For this review, take the finished solid that the model builds, in its own axes (mm). A direction names the side the tool comes from. Coordinates: 2 decimals unless noted, no trailing zeros. Order: outer loops, then holes, each group sorted by start corner. A loop starts at its lowest first (then second) coordinate and runs counter-clockwise, first axis right, second up. Notation, with made-up numbers: (-22.5, 45) -> (-5.5, 45) arc R32 cw to (-5.5, 80) -> close; hole circle Ø10 at (74, 16). An arc over 180 degrees is marked (long way). Answer as a JSON object with one key per item and string values. Group by question number.
1) Machinability: for faces 1 (the flat face through (7, 0, 15)), 2 (the flat face through (-7, 0, 15)), 3 (the flat face through (0, -7, 15)), 4 (the flat face through (-0.1, 5.4, 0)), 5 (the flat face through (0, 0, 18)), which of the approach directions +Z, -Z, +X, -X, +Y, -Y give a long, thin tool a straight path to every point of the face, cutting with its end or side? Answer none if there is none.
2) Wall thickness on L1, parallel to X at y = -3.5, z = 6.25; L2, parallel to X at y = 3, z = 10.5: over which ranges is each line inside the solid? List them lowest first.
3) For pin 1 (8 mm diameter, centred on x = -4, y = 5, fed in from -Z); pin 2 (8 mm diameter, centred on x = -1.5, z = 14.5, fed in from +Y); pin 3 (1 mm diameter, centred on y = 1, z = 13.5, fed in from +X); pin 4 (3 mm diameter, centred on y = 2, z = 15.5, fed in from -X), all flat-tipped, find the tip position at first contact; note any pin that passes through.
4) Draft analysis for pull direction X (two halves, no side actions). For faces 6 (the flat face through (5, 0, 9)), 7 (the flat face through (-8, 0, 5)), 8 (the flat face through (0, 7, 15)), state which applies: +X half, -X half, draft (parallel to the pull), parting line (faces both ways), or undercut.
5) Add section D-D, the plane z = 17.25. Write out the cut boundary in (x, y), then the cut area to 3 significant figures.
6) Add section B-B, the plane x = 2.25. Write out the cut boundary in (y, z).
7) Add section A-A, the plane z = 8. Write out the cut boundary in (x, y), then the cut area to 3 significant figures.
from build123d import *

# Parameters (mm, degrees)
BOX002_W     = 10
BOX002_H     = 10
BOX002_DEPTH = 18
BOX001_W     = 14
BOX001_H     = 14
BOX001_DEPTH = 10
BOX_W        = 16
BOX_H        = 16
BOX_DEPTH    = 10


with BuildPart() as cube002:
    # Box002 → Box002 (new body)
    with BuildSketch(Plane(origin=(-5, -5, 0), x_dir=(1, 0, 0), z_dir=(0, 0, 1))):
        with Locations((5, 5)):
            Rectangle(BOX002_W, BOX002_H)
    extrude(amount=BOX002_DEPTH)


with BuildPart() as cube001:
    # Box001 → Box001 (new body)
    with BuildSketch(Plane(origin=(-7, -7, 10), x_dir=(1, 0, 0), z_dir=(0, 0, 1))):
        with Locations((7, 7)):
            Rectangle(BOX001_W, BOX001_H)
    extrude(amount=BOX001_DEPTH)


with BuildPart() as cut:
    # Box → Box (new body)
    with BuildSketch(Plane(origin=(-8, -8, 0), x_dir=(1, 0, 0), z_dir=(0, 0, 1))):
        with Locations((8, 8)):
            Rectangle(BOX_W, BOX_H)
    extrude(amount=BOX_DEPTH)

    # Fusion: union Cube001
    add(cube001.part)

    # Cut: cut Cube002
    add(cube002.part, mode=Mode.SUBTRACT)


solid = cut.part
Output values:
{
 "1": {"face 1": "+Z, +X, +Y, -Y", "face 2": "+Z, -X, +Y, -Y", "face 3": "+Z, +X, -X, -Y", "face 4": "-Z, +X, -X, +Y, -Y", "face 5": "-Z"},
 "2": {"L1": "x = -8 to -5, 5 to 8", "L2": "x = -7 to -5, 5 to 7"},
 "3": {"pin 1": "stops at z = 0", "pin 2": "stops at y = 7", "pin 3": "stops at x = 7", "pin 4": "stops at x = -7"},
 "4": {"face 6": "undercut", "face 7": "-X half", "face 8": "draft"},
 "5": {"outline": "(-7, -7) -> (7, -7) -> (7, 7) -> (-7, 7) -> close; hole (-5, -5) -> (5, -5) -> (5, 5) -> (-5, 5) -> close", "area": "96.0 mm²"},
 "6": {"outline": "(-8, 0) -> (-5, 0) -> (-5, 18) -> (5, 18) -> (5, 0) -> (8, 0) -> (8, 10) -> (7, 10) -> (7, 20) -> (-7, 20) -> (-7, 10) -> (-8, 10) -> close"},
 "7": {"outline": "(-8, -8) -> (8, -8) -> (8, 8) -> (-8, 8) -> close; hole (-5, -5) -> (5, -5) -> (5, 5) -> (-5, 5) -> close", "area": "156 mm²"}
}
